```python
from build123d import *

# Parameters (mm, degrees)
IZIM1_R                     = 7.5
Y_KSEKLIK_EKSTR_ZYON1_DEPTH = 331
IZIM2_R                     = 14.25
Y_KSEKLIK_EKSTR_ZYON2_DEPTH = 2
RADYUS1_R                   = 1
IZIM6_R                     = 5
KES_EKSTR_ZYON1_DEPTH       = 22


with BuildPart() as part:
    # Çizim1 → Yükseklik-Ekstrüzyon1 (new body)
    with BuildSketch(Plane.XY):
        Circle(IZIM1_R)
    extrude(amount=Y_KSEKLIK_EKSTR_ZYON1_DEPTH)

    # Çizim2 → Yükseklik-Ekstrüzyon2 (add)
    with BuildSketch(Plane.XY.offset(331)):
        Circle(IZIM2_R)
    extrude(amount=Y_KSEKLIK_EKSTR_ZYON2_DEPTH)

    # Radyus1
    radyus1_edges = [part.edges().sort_by_distance(p)[0] for p in [
        (-14.25, 0, 333),
    ]]
    fillet(radyus1_edges, radius=RADYUS1_R)

    # Çizim6 → Kes-Ekstrüzyon1 (cut, symmetric)
    with BuildSketch(Plane(origin=(0, 0, 0), x_dir=(0, 0, -1), z_dir=(1, 0, 0))):
        with Locations((-10, 0)):
            Circle(IZIM6_R)
    extrude(amount=KES_EKSTR_ZYON1_DEPTH, both=True, mode=Mode.SUBTRACT)


solid = part.part
```
Read the model definition and answer for the solid it produces. Units are mm, in the model's axes. A direction names the side the tool comes from. Coordinates: 2 decimals unless noted, no trailing zeros. Order: outer loops, then holes, each group sorted by start corner. A loop starts at its lowest first (then second) coordinate and runs counter-clockwise, first axis right, second up. Notation, with made-up numbers: (4.5, 74) - (17.5, 74) arc R17 cw to (17.5, 83) - close; hole circle Ø2 at (72, 45.5). An arc over 180 degrees is marked (long way). Answer as a JSON object with one key per item and string values. Group by question number.
Item 1: Section C-C (z = 10) is taken. Give the vertices of the cut face in (x, y).
Item 2: A tool of negligible diameter and unlimited length cuts with its end or side. For faces 1 (the face through (13.163, -5.458, 331.493)), 2 (the face through (6, -6, 331)), from which of +Z, -Z, +X, -X, +Y, -Y can it reach the whole face along a straight path? Write none if from no direction.
Item 3: Section D-D (z = 255) is taken. Give the vertices of the cut face in (x, y).
Item 4: Consider probe 1 along Z at (x, y) = (-4, 0); probe 2 along Z at (x, y) = (6, -9); probe 3 along Z at (x, y) = (-6.5, -3). Determine where each line is inside the solid, lowest interval first. Write a range as from..to.
Item 5: Section B-B (y = 0) is taken. Give the vertices of the cut face in (x, z), plus the area to 3 significant figures.
Item 6: Section A-A (x = 0) is taken. Give the vertices of the cut face in (y, z).
Item 7: The mould has two halves that part along Y. Classify faces 3 (the face through (0, -3, 14)), 4 (the face through (-7.493, 0.33, 163.183)), 5 (the face through (0, 0, 333)): +Y half, -Y half, draft (parallel to the pull), parting line (faces both ways), or undercut.
Item 8: Flat-ended cylindrical pins translate along their axes: P1, Ø8, axis at x = 2, z = 77.5, coming from the -Y side; P2, Ø1.5, axis at y = 1, z = 290.5, coming from the -X side; P3, Ø10, axis at x = 5, y = 9, coming from the -Z side; P4, Ø4, axis at x = 8.5, y = -7, coming from the -Z side. Find the tip coordinate at first contact, or state that the pin passes through.
Results are:
{
 "1": {"outline": "(-5.59, -5) arc R7.5 ccw to (5.59, -5) - close; (-5.59, 5) - (5.59, 5) arc R7.5 ccw to start"},
 "2": {"face 1": "+Z, -Z", "face 2": "-Z"},
 "3": {"outline": "circle Ø15 at (0, 0)"},
 "4": {"probe 1": "z = 0..5, 15..333", "probe 2": "z = 331..333", "probe 3": "z = 0..6, 14..333"},
 "5": {"outline": "(-14.25, 331) - (-7.5, 331) - (-7.5, 15) - (7.5, 15) - (7.5, 331) - (14.25, 331) - (14.25, 332) arc R1 ccw to (13.25, 333) - (-13.25, 333) arc R1 ccw to (-14.25, 332) - close; (-7.5, 0) - (7.5, 0) - (7.5, 5) - (-7.5, 5) - close", "area": "4,870 mm^2"},
 "6": {"outline": "(-14.25, 331) - (-7.5, 331) - (-7.5, 0) - (7.5, 0) - (7.5, 331) - (14.25, 331) - (14.25, 332) arc R1 ccw to (13.25, 333) - (-13.25, 333) arc R1 ccw to (-14.25, 332) - close; hole circle Ø10 at (0, 10)"},
 "7": {"face 3": "undercut", "face 4": "parting line", "face 5": "draft"},
 "8": {"P1": "stops at y = -7.5", "P2": "stops at x = -7.5", "P3": "stops at z = 0", "P4": "stops at z = 331"}
}
